Part print with two shaded views. Sizes in mm from the minimum x, y, z corner. A direction names the side the tool comes from. Give positions to 0.01 mm unless a question says otherwise; leave off trailing zeros. Write each loop counter-clockwise with the first axis right and the second up, starting at its lowest first coordinate (ties: lowest second). Pieces come first, ordered by that corner, then holes.
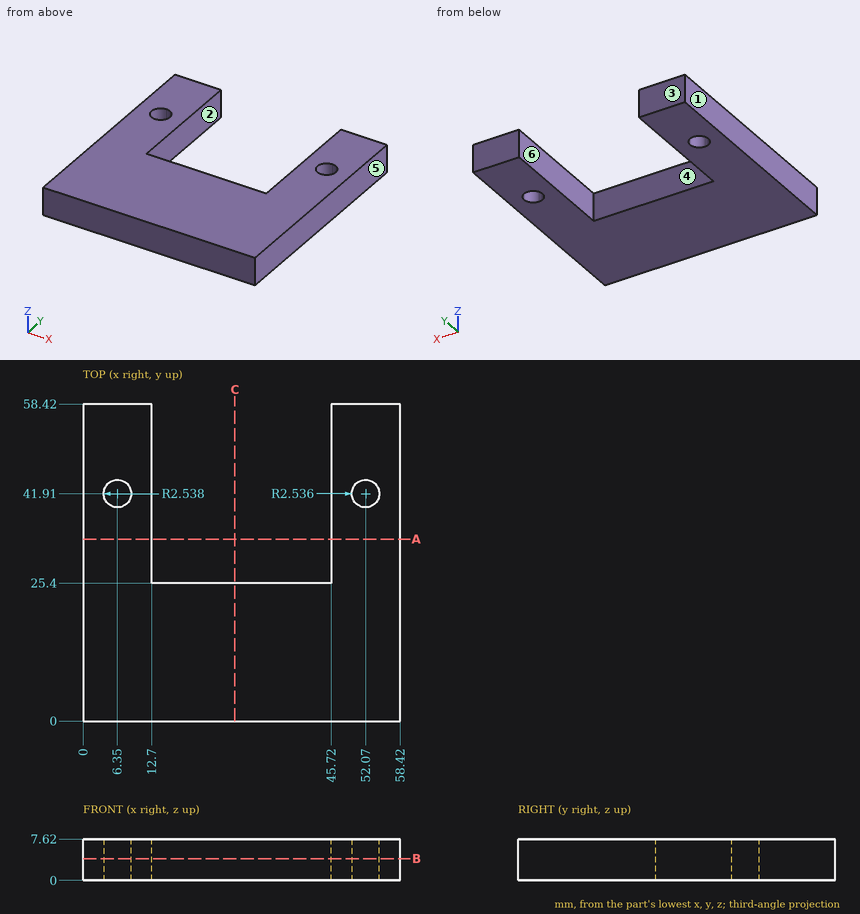
1) Saw through at B-B, the plane z = 4. Write the cut outline in (x, y), then the cut area to 3 significant figures.
Answers follow:
outline: (0, 0) - (58.42, 0) - (58.42, 58.42) - (45.72, 58.42) - (45.72, 25.4) - (12.7, 25.4) - (12.7, 58.42) - (0, 58.42) - close; hole circle Ø5.08 at (6.35, 41.91); hole circle Ø5.07 at (52.07, 41.91)
area: 2,280 mm2
2) Saw through at C-C, the plane x = 28. Write the cut outline in (y, z), then the cut area to 3 significant figures.
Answers follow:
outline: (0, 0) - (25.4, 0) - (25.4, 7.62) - (0, 7.62) - close
area: 194 mm2
3) 3-axis set-ups, long thin cutter, end or side, ignore diameter. For the marked faces 5 and 6: which of +Z, -Z, +X, -X, +Y, -Y reach the whole face in a straight line?
Answers follow:
face 5: +Z, -Z, +X, +Y, -Y
face 6: +Z, -Z, +Y
4) Wall check: L1, parallel to X at y = 47.5, z = 3.75; L2, parallel to Y at x = 22, z = 2; L3, parallel to X at y = 41, z = 1. Give the ranges that are in metal, low to high.
Answers follow:
L1: x = 0 to 12.7, 45.72 to 58.42
L2: y = 0 to 25.4
L3: x = 0 to 3.98, 8.72 to 12.7, 45.72 to 49.7, 54.44 to 58.42
5) Two-plate mould, pull along X, no slides. Class the marked faces 1, 2, 3 and 4: +X half, -X half, draft (parallel to the pull), parting line (faces both ways), or undercut.
Answers follow:
face 1: -X half
face 2: undercut
face 3: draft
face 4: undercut
6) Saw through at A-A, the plane y = 33.5. Write the cut outline in (x, z), then the cut area to 3 significant figures.
Answers follow:
outline: (0, 0) - (12.7, 0) - (12.7, 7.62) - (0, 7.62) - close; (45.72, 0) - (58.42, 0) - (58.42, 7.62) - (45.72, 7.62) - close
area: 194 mm2
